```python
from build123d import *

# Parameters (mm, degrees)
SKETCH1_W            = 100
SKETCH1_H            = 100
BOSS_EXTRUDE1_DEPTH  = 180
SKETCH2_R            = 34.257790197
BOSS_EXTRUDE2_DEPTH  = 350
SKETCH3_W            = 152.006357392
SKETCH3_H            = 282.452416457
CUT_EXTRUDE2_DEPTH   = 400
CUT_EXTRUDE3_DEPTH   = 400
CUT_EXTRUDE4_DEPTH   = 400
CUT_EXTRUDE5_DEPTH   = 400
SKETCH7_W            = 160.159381639
SKETCH7_H            = 147.362276113
CUT_EXTRUDE6_DEPTH   = 400
SKETCH8_W            = 147.310744502
SKETCH8_H            = 162.038906966
CUT_EXTRUDE7_DEPTH   = 400
SKETCH9_R            = 31.847293423
CUT_EXTRUDE8_DEPTH   = 400
SKETCH10_W           = 140.220962397
SKETCH10_H           = 212.033531124
CUT_EXTRUDE9_DEPTH   = 400
SKETCH11_R           = 13.603137886
CUT_EXTRUDE11_DEPTH  = 15
SKETCH12_R           = 12.495422516
BOSS_EXTRUDE3_DEPTH  = 15
SKETCH13_R           = 1.594865099
BOSS_EXTRUDE4_DEPTH  = 4
SKETCH14_W           = 100.74862993
SKETCH14_H           = 110.555003588
CUT_EXTRUDE13_DEPTH  = 400
BOSS_EXTRUDE5_DEPTH  = 1
SKETCH16_W           = 24.504230724
SKETCH16_H           = 30.458347221
BOSS_EXTRUDE6_DEPTH  = 5
SKETCH17_W           = 18.669530869
SKETCH17_H           = 22.4027039
BOSS_EXTRUDE7_DEPTH  = 1
SKETCH18_W           = 4.907623399
SKETCH18_H           = 5.170746831
SKETCH18_W_2         = 3.981473695
SKETCH18_H_2         = 5.451349552
BOSS_EXTRUDE8_DEPTH  = 1
BOSS_EXTRUDE9_DEPTH  = 1
SKETCH21_W           = 16.281298494
SKETCH21_H           = 30.70477752
BOSS_EXTRUDE10_DEPTH = 5
SKETCH22_W           = 0.561666562
SKETCH22_H           = 0.603858724
SKETCH22_W_2         = 0.53443704
SKETCH22_W_3         = 0.536755884
SKETCH22_H_2         = 0.595744993
SKETCH22_W_4         = 0.555081497
SKETCH22_H_3         = 0.603543747
SKETCH22_H_4         = 0.606016701
SKETCH22_W_5         = 0.51195437
BOSS_EXTRUDE11_DEPTH = 1


with BuildPart() as part:
    # Sketch1 → Boss-Extrude1 (new body)
    with BuildSketch(Plane(origin=(0, 0, 0), x_dir=(1, 0, 0), z_dir=(0, 1, 0))):
        with Locations((-50, 50)):
            Rectangle(SKETCH1_W, SKETCH1_H)
    extrude(amount=BOSS_EXTRUDE1_DEPTH)

    # Sketch2 → Boss-Extrude2 (add, symmetric)
    with BuildSketch(Plane(origin=(0, 180, 0), x_dir=(1, 0, 0), z_dir=(0, 1, 0))):
        with Locations(Location((-51.377291833, 49.076536384, 0), (0, 0, 270))):
            Circle(SKETCH2_R)
    extrude(amount=BOSS_EXTRUDE2_DEPTH, both=True)

    # Sketch3 → Cut-Extrude2 (cut)
    with BuildSketch(Plane(origin=(0, 0, 0), x_dir=(0, 0, -1), z_dir=(1, 0, 0))):
        with Locations((57.419900112, 502.274302507)):
            Rectangle(SKETCH3_W, SKETCH3_H)
    extrude(amount=-CUT_EXTRUDE2_DEPTH, mode=Mode.SUBTRACT)

    # Sketch4 → Cut-Extrude3 (cut)
    with BuildSketch(Plane(origin=(0, 0, 0), x_dir=(0, 0, -1), z_dir=(1, 0, 0))):
        Polygon((12.981970869, 0), (-8.994244796, 25.828096003), (-18.564506014, -15.259465835), align=None)
        Polygon((85.072517936, -1.448103984), (109.237639161, 19.113145112), (115.920034239, -3.267382694), align=None)
        Polygon((12.981970869, 180), (-8.994244796, 148.537596011), (-15.418178585, 193.219274892), align=None)
        Polygon((85.072517936, 181.854312784), (103.841225373, 159.795920888), (106.132549481, 198.647393934), align=None)
    extrude(amount=-CUT_EXTRUDE3_DEPTH, mode=Mode.SUBTRACT)

    # Sketch5 → Cut-Extrude4 (cut)
    with BuildSketch(Plane.XY):
        Polygon((-85.623287335, 0), (-106.370377984, 21.426392531), (-122.288861874, 3.209259887), (-93.526345261, -19.884701759), align=None)
        Polygon((-15.694988751, 0), (0, 15.257385304), (12.122677088, 15.257385304), (10.563067769, -19.884701759), align=None)
        Polygon((-87.166490339, 180.248071029), (-106.370377984, 151.29108453), (-117.705469457, 200.501115102), align=None)
        Polygon((-15.694988751, 180.248071029), (7.833767065, 153.279557508), (0, 193.941208308), align=None)
    extrude(amount=-CUT_EXTRUDE4_DEPTH, mode=Mode.SUBTRACT)

    # Sketch6 → Cut-Extrude5 (cut)
    with BuildSketch(Plane(origin=(0, 180, 0), x_dir=(1, 0, 0), z_dir=(0, 1, 0))):
        Polygon((-112.386997555, 28.400400964), (-64.261264503, -10.212759359), (-84.406366528, -15.51192827), (-124.649689542, -15.51192827), align=None)
        Polygon((-97.065537028, 135.861756084), (-119.37552445, 77.792688888), (-118.043343626, 64.347606737), (-66.428694172, 110.575168787), align=None)
        Polygon((-24.69640689, -21.815840769), (11.092108798, -8.97361337), (17.428316417, 32.393768119), (-38.531576846, -11.139157378), align=None)
        Polygon((-17.445484601, 140.804394854), (35.417473102, 107.262520599), (9.305452855, 72.996438725), (-31.724385352, 103.625272537), align=None)
    extrude(amount=-CUT_EXTRUDE5_DEPTH, mode=Mode.SUBTRACT)

    # Sketch7 → Cut-Extrude6 (cut)
    with BuildSketch(Plane.XY):
        with Locations((-66.123258915, -136.36252694)):
            Rectangle(SKETCH7_W, SKETCH7_H)
    extrude(amount=-CUT_EXTRUDE6_DEPTH, mode=Mode.SUBTRACT)

    # Sketch8 → Cut-Extrude7 (cut)
    with BuildSketch(Plane.XY):
        with Locations((-53.541153336, 332.448287589)):
            Rectangle(SKETCH8_W, SKETCH8_H)
    extrude(amount=-CUT_EXTRUDE7_DEPTH, mode=Mode.SUBTRACT)

    # Sketch9 → Cut-Extrude8 (cut)
    with BuildSketch(Plane(origin=(0, 251.428834106, 0), x_dir=(1, 0, 0), z_dir=(0, 1, 0))):
        with Locations(Location((-50.808993157, 49.032036374, 0), (0, 0, 270))):
            Circle(SKETCH9_R)
    extrude(amount=-CUT_EXTRUDE8_DEPTH, mode=Mode.SUBTRACT)

    # Sketch10 → Cut-Extrude9 (cut)
    with BuildSketch(Plane.ZY.offset(100)):
        with Locations((14.299084536, 180.100625535)):
            Rectangle(SKETCH10_W, SKETCH10_H)
    extrude(amount=-CUT_EXTRUDE9_DEPTH, mode=Mode.SUBTRACT)

    # Sketch11 → Cut-Extrude11 (cut)
    with BuildSketch(Plane.ZY.offset(100)):
        with Locations((-50.413251954, 76.264646142)):
            Circle(SKETCH11_R)
    extrude(amount=-CUT_EXTRUDE11_DEPTH, mode=Mode.SUBTRACT)

    # Sketch12 → Boss-Extrude3 (add)
    with BuildSketch(Plane.ZY.offset(85)):
        with Locations(Location((-50.658800768, 76.222522328, 0), (0, 0, 114.353089558))):
            Circle(SKETCH12_R)
    extrude(amount=BOSS_EXTRUDE3_DEPTH)

    # Sketch13 → Boss-Extrude4 (add)
    with BuildSketch(Plane(origin=(-85, 0, 0), x_dir=(0, 0, -1), z_dir=(1, 0, 0))):
        with Locations(Location((49.945205578, 75.944780088, 0), (0, 0, 180))):
            Circle(SKETCH13_R)
    extrude(amount=BOSS_EXTRUDE4_DEPTH)

    # Sketch14 → Cut-Extrude13 (cut)
    with BuildSketch(Plane.ZY.offset(100)):
        with Locations((-65.350029467, 250.603414818)):
            Rectangle(SKETCH14_W, SKETCH14_H)
    extrude(amount=-CUT_EXTRUDE13_DEPTH, mode=Mode.SUBTRACT)

    # Sketch15 → Boss-Extrude5 (add)
    with BuildSketch(Plane.ZY.offset(100)):
        Polygon((-18.461827727, 14.847435435), (-80.507743362, 14.847435435), (-80.507743362, 160.896793159), (-55.811396663, 160.896793159), (-55.811396663, 74.083859973), (-18.461827727, 74.083859973), align=None)
    extrude(amount=BOSS_EXTRUDE5_DEPTH)

    # Sketch16 → Boss-Extrude6 (add)
    with BuildSketch(Plane.ZY.offset(101)):
        with Locations((-39.275145749, 45.136437142)):
            Rectangle(SKETCH16_W, SKETCH16_H)
    extrude(amount=BOSS_EXTRUDE6_DEPTH)

    # Sketch17 → Boss-Extrude7 (add)
    with BuildSketch(Plane.ZY.offset(101)):
        with Locations((-67.04663872, 130.409241603)):
            Rectangle(SKETCH17_W, SKETCH17_H)
    extrude(amount=BOSS_EXTRUDE7_DEPTH)

    # Sketch18 → Boss-Extrude8 (add)
    with BuildSketch(Plane.ZY.offset(102)):
        with Locations((-71.625108618, 130.213401885)):
            Rectangle(SKETCH18_W, SKETCH18_H)
        with Locations((-62.297675883, 129.867186512)):
            Rectangle(SKETCH18_W_2, SKETCH18_H_2)
    extrude(amount=BOSS_EXTRUDE8_DEPTH)

    # Sketch19 → Boss-Extrude9 (add)
    with BuildSketch(Plane.ZY.offset(102)):
        Polygon((-66.976455081, 134.868836652), (-73.7929295, 134.868836652), (-73.7929295, 134.108269479), (-74.571872104, 134.108269479), (-74.571872104, 140.512729543), (-73.7929295, 140.512729543), (-72.165965418, 140.512729543), (-72.233411796, 137.421948277), (-71.48458153, 137.421948277), (-71.410861795, 140.512729543), (-69.158339735, 140.504865112), (-69.158339735, 137.421948277), (-68.22174926, 137.421948277), (-68.22174926, 140.567922793), (-65.426885805, 140.567922793), (-65.515241968, 137.446210948), (-64.714122339, 137.446210948), (-64.714122339, 140.567922793), (-62.410871788, 140.567922793), (-62.410871788, 137.210126003), (-61.403493639, 137.210126003), (-61.403493639, 140.631129361), (-58.889974549, 140.631129361), (-58.889974549, 136.595539338), (-59.698319644, 136.595539338), (-59.698319644, 139.99489006), (-60.695848378, 139.984078324), (-60.695848378, 136.667717235), (-63.090112056, 136.667717235), (-63.090112056, 139.979723883), (-64.00479018, 139.979723883), (-64.00479018, 136.667717235), (-66.334605538, 136.667717235), (-66.334605538, 139.902697072), (-67.48995239, 139.902697072), (-67.48995239, 136.667717235), (-70.008746759, 136.667717235), (-70.008746759, 139.902697072), (-70.709698815, 139.902697072), (-70.783897489, 136.693128041), (-72.921241048, 136.693128041), (-72.921241048, 139.545601992), (-73.7929295, 139.545601992), (-73.7929295, 135.423339258), (-66.976455081, 135.49721976), align=None)
    extrude(amount=BOSS_EXTRUDE9_DEPTH)

    # Sketch21 → Boss-Extrude10 (add)
    with BuildSketch(Plane.ZY.offset(101)):
        with Locations((-60.112791098, 44.859291254)):
            Rectangle(SKETCH21_W, SKETCH21_H)
    extrude(amount=BOSS_EXTRUDE10_DEPTH)

    # Sketch22 → Boss-Extrude11 (add)
    with BuildSketch(Plane.ZY.offset(102)):
        with Locations((-60.80943011, 132.899150377)):
            Rectangle(SKETCH22_W, SKETCH22_H)
        with Locations((-61.69225831, 132.899150377)):
            Rectangle(SKETCH22_W_2, SKETCH22_H)
        with Locations((-62.62493976, 132.903207243)):
            Rectangle(SKETCH22_W_3, SKETCH22_H_2)
        with Locations((-63.54978292, 132.899150377)):
            Rectangle(SKETCH22_W_4, SKETCH22_H)
        with Locations((-60.80943011, 126.809637752)):
            Rectangle(SKETCH22_W, SKETCH22_H_3)
        with Locations((-61.69225831, 126.810874229)):
            Rectangle(SKETCH22_W_2, SKETCH22_H_4)
        with Locations((-62.612539003, 126.810874229)):
            Rectangle(SKETCH22_W_5, SKETCH22_H_4)
        with Locations((-63.54978292, 126.810874229)):
            Rectangle(SKETCH22_W_4, SKETCH22_H_4)
    extrude(amount=BOSS_EXTRUDE11_DEPTH)


solid = part.part
```
The listing builds one solid part. Answer for the finished solid, in the listing's coordinates (mm). A direction names the side the tool comes from. Coordinates: 2 decimals unless noted, no trailing zeros. Write each loop counter-clockwise with the first axis right and the second up, starting at its lowest first coordinate (ties: lowest second). Pieces come first, ordered by that corner, then holes. Notation, with made-up numbers: (-18, 7) - (-12, 7) arc R23 ccw to (-12, 31) - close; hole circle Ø6 at (34, 26.25). An arc over 180 degrees is marked (long way). Return JSON: item names as keys, results as strings. Group by question number.
1. A cutting plane is placed at A-A, the plane x = -40. Determine the outline of the cut face in (y, z).
2. Given pin 1 (0.5 mm diameter, centred on x = -102.5, y = 137.5, fed in from +Z); pin 2 (0.7 mm diameter, centred on x = -102.5, y = 133, fed in from -Z); pin 3 (1.1 mm diameter, centred on x = -102.5, y = 130.5, fed in from -Z); pin 4 (8 mm diameter, centred on y = -21, z = -88, fed in from +X), each flat-ended and moving along its own axis, determine where each tip first touches the part or whether it passes through.
3. A cutting plane is placed at C-C, the plane x = -6.5. Determine the outline of the cut face in (y, z), plus the area to 3 significant figures.
4. A cutting plane is placed at B-B, the plane x = -74.5. Determine the outline of the cut face in (y, z).
5. Which of the six approach directions +Z, -Z, +X, -X, +Y, -Y give full straight-line access (tool end or side, diameter ignored) to faces 1 (the flat face through (-52, 180, -85)), 2 (the flat face through (-103, 60.366, -39)), 3 (the flat face through (-85, 65, -57)), 4 (the flat face through (-103, 45, -27.023)), 5 (the flat face through (-11.937, 39.458, -9.55))?
6. Determine the mould class of faces 6 (the flat face through (-103, 45, -51.972)), 7 (the cylindrical face through (-84.82, -30.9, -56.5)), 8 (the flat face through (-82, -62.681, -57)), 9 (the flat face through (-53, 87, -100)) for opening direction Z: released by +Z, released by -Z, zero draft, split by the parting line, or undercut.
7. A cutting plane is placed at D-D, the plane z = -7. Determine the outline of the cut face in (x, y).
8. Straight lines are drawn through the part: L1, parallel to Z at x = -51, y = 45; L2, parallel to Z at x = -100, y = 100; L3, parallel to Y at x = -29, z = -24. For each, find the intervals that lie inside material, in ascending order.
Ans:
{
 "1": {"outline": "(-62.68, -81.39) - (0, -81.39) - (0, -86.77) - (11.25, -100) - (164.31, -100) - (180, -86.65) - (180, -81.39) - (195.33, -81.39) - (195.33, -78.99) - (-62.68, -78.99) - close; (-62.68, -19.08) - (74.08, -19.08) - (74.08, 0) - (15.26, 0) - (0, -12.98) - (0, -16.76) - (-62.68, -16.76) - close"},
 "2": {"pin 1": "z = -58.89", "pin 2": "z = -74.08", "pin 3": "z = -76.38", "pin 4": "through"},
 "3": {"outline": "(8.94, -84.8) - (169.71, -84.8) - (169.71, -55.81) - (74.08, -55.81) - (74.08, -13.78) - (8.94, -13.78) - close", "area": "7,400 mm²"},
 "4": {"outline": "(-62.68, -74.35) - (0, -74.35) - (0, -86.77) - (11.25, -100) - (164.31, -100) - (180, -86.65) - (180, -74.35) - (195.33, -74.35) - (195.33, -70.32) - (-62.68, -70.32) - close; (-62.68, -27.75) - (74.08, -27.75) - (74.08, 0) - (15.26, 0) - (0, -12.98) - (0, -23.8) - (-62.68, -23.8) - close"},
 "5": {"face 1": "-Z, +Y", "face 2": "+Z, -Z, -X, +Y", "face 3": "none", "face 4": "+Z, -X, +Y, -Y", "face 5": "+Z, +X, +Y, -Y"},
 "6": {"face 6": "undercut", "face 7": "split by the parting line", "face 8": "zero draft", "face 9": "released by -Z"},
 "7": {"outline": "(-85.71, 7.03) - (-15.21, 7.03) - (-15.21, 74.08) - (-85.71, 74.08) - close"},
 "8": {"L1": "-100 to -80.88, -17.19 to 0", "L2": "-80.51 to -55.81", "L3": "-62.68 to 74.08"}
}
